```python
from build123d import *

# Parameters (mm, degrees)
SKETCH1_R           = 2.794
SKETCH1_R_2         = 1.5875
BOSS_EXTRUDE1_DEPTH = 165.1
BOSS_EXTRUDE2_DEPTH = 1.27


with BuildPart() as part:
    # Sketch1 → Boss-Extrude1 (new body)
    with BuildSketch(Plane(origin=(0, 0, 0), x_dir=(1, 0, 0), z_dir=(0, 1, 0))):
        Circle(SKETCH1_R)
        Circle(SKETCH1_R_2, mode=Mode.SUBTRACT)
    extrude(amount=BOSS_EXTRUDE1_DEPTH)

    # Sketch2 → Boss-Extrude2 (add)
    with BuildSketch(Plane(origin=(0, 6.35, 0), x_dir=(-1, 0, 0), z_dir=(0, -1, 0))):
        with BuildLine():
            Line((-3.991923346, -0.762), (-2.688083332, -0.762))
            ThreePointArc((-2.688083332, -0.762), (0, -2.794), (2.688083332, -0.762))
            Line((2.688083332, -0.762), (3.991923346, -0.762))
            ThreePointArc((3.991923346, -0.762), (0, -4.064), (-3.991923346, -0.762))
        make_face()
    boss_extrude2 = extrude(amount=-BOSS_EXTRUDE2_DEPTH)

    # Mirror1: Boss-Extrude2 across plane
    add(boss_extrude2.mirror(Plane(origin=(0, 82.55, 0), x_dir=(0, 0, 1), z_dir=(0, -1, 0))))


solid = part.part
```
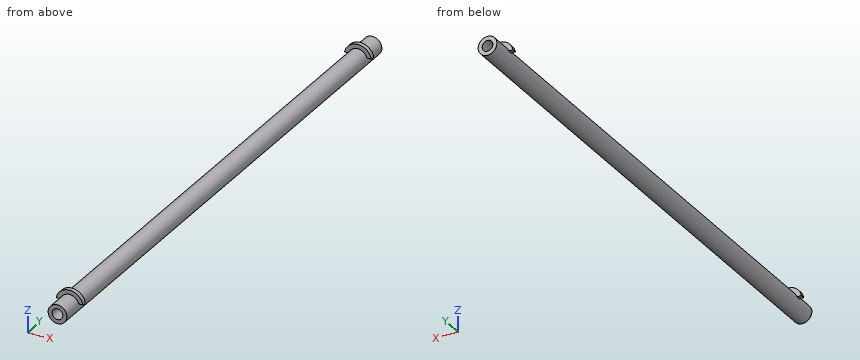
Work out the finished part from the listing and answer in its coordinate system (mm). Round coordinates to 2 decimals unless told otherwise and drop trailing zeros. Write each loop counter-clockwise with the first axis right and the second up, starting at its lowest first coordinate (ties: lowest second). Pieces come first, ordered by that corner, then holes.
1) A cutting plane is placed at B-B on y = 90. Determine the outline of the cut face in (x, z) (1 decimal).
2) Consider probe 1 along Y at (x, z) = (3.5, 2); probe 2 along Z at (x, y) = (0, 51.5). Determine where each line is inside the solid, lowest interval first.
3) A cutting plane is placed at A-A on x = 0. Determine the outline of the cut face in (y, z).
4) Flat-ended cylindrical pins translate along their axes: P1, Ø1, axis at x = 3, y = 158, coming from the -Z side; P2, Ø3, axis at y = 30.5, z = -2, coming from the -X side; P3, Ø2, axis at x = -2.5, y = 144.5, coming from the +Z side; P4, Ø3, axis at x = 0, z = 0, coming from the +Y side. Find the tip coordinate at first contact, or state that the pin passes through.
Entries:
1. outline: circle Ø5.6 at (0, 0); hole circle Ø3.2 at (0, 0)
2. probe 1: y = 6.35 to 7.62, 157.48 to 158.75
2. probe 2: z = -2.79 to -1.59, 1.59 to 2.79
3. outline: (0, -2.79) - (165.1, -2.79) - (165.1, -1.59) - (0, -1.59) - close; (0, 1.59) - (165.1, 1.59) - (165.1, 2.79) - (158.75, 2.79) - (158.75, 4.06) - (157.48, 4.06) - (157.48, 2.79) - (7.62, 2.79) - (7.62, 4.06) - (6.35, 4.06) - (6.35, 2.79) - (0, 2.79) - close
4. P1: stops at z = -1.25
4. P2: stops at x = -2.75
4. P3: stops at z = 2.36
4. P4: passes through
